Input: part model. Units: mm. Frame: model coordinates. A direction names the side the tool comes from. Round coordinates to 2 decimals unless told otherwise and drop trailing zeros. Loops run counter-clockwise (first coordinate to the right, second up) from the corner with the lowest first, then second, coordinate; pieces in that order, holes last. Notation, with made-up numbers: M -14.75,16 L 43.25,16 A16 ccw 43.25,20 Z; hole C 53.5,-21 d11. An arc over 180 degrees is marked long. Put each result on its own line as item: value. Start each with the question number.
1) Draft query along X for faces 6 (the face through (-1.5, -3, 0)), 7 (the face through (13, 4, -3)), 8 (the face through (21.4, -0.2, -0.5)). Return one class per face: +X half, -X half, draft (parallel to the pull), parting line (faces both ways), or undercut.
2) Line query: probe 1 along X at (y, z) = (-4.75, 3); probe 2 along X at (y, z) = (-1, -3); probe 3 along X at (y, z) = (8.75, -2.25). Output: solid intervals per line, ascending.
3) Section A-A on y = -1.3. State how many separate pieces and enclosed holes the cut face has, plus the area to 3 significant figures.
4) Section D-D on z = 4.75. Output: boundary loops of the cut face in (x, y).
5) Section C-C on z = 0.5. Output: boundary loops of the cut face in (x, y), plus the area to 3 significant figures.
6) Section B-B on x = 18.5. Output: boundary loops of the cut face in (y, z).
7) Reachability of faces 1 (the face through (0, -6, 4)), 2 (the face through (-6.2, -3, 0)), 3 (the face through (0, 10, -4)), 4 (the face through (19, 3.4, 3)), 5 (the face through (-9, 0, 0)) from +Z, -Z, +X, -X, +Y, -Y: full face, straight path, thin tool, end or side. Return the list, or none.
8) Pin query (flat end, axial travel): pin 1 (3.5 mm diameter, centred on y = 1.5, z = -2.5, fed in from +X); pin 2 (6.5 mm diameter, centred on y = -4, z = -1.5, fed in from +X); pin 3 (2.5 mm diameter, centred on x = 2.5, z = -1, fed in from +Y); pin 4 (2.5 mm diameter, centred on x = 20, y = -3, fed in from -Z). Return the tip coordinate at first contact, or that it passes through.
from build123d import *

# Parameters (mm, degrees)
SKETCH2_W           = 26
SKETCH2_H           = 11
SKETCH2_W_2         = 20.4
SKETCH2_H_2         = 6.5
BOSS_EXTRUDE1_DEPTH = 10
SKETCH3_W           = 26
SKETCH3_H           = 11
SKETCH3_W_2         = 2.5
SKETCH3_H_2         = 6.5
BOSS_EXTRUDE2_DEPTH = 6
SKETCH4_W           = 11
SKETCH4_H           = 9.4
SKETCH4_R           = 2.85
BOSS_EXTRUDE3_DEPTH = 6
FILLET1_R           = 2


with BuildPart() as part:
    # Sketch2 → Boss-Extrude1 (new body)
    with BuildSketch(Plane(origin=(0, 0, 0), x_dir=(1, 0, 0), z_dir=(0, 1, 0))):
        Rectangle(SKETCH2_W, SKETCH2_H)
        Rectangle(SKETCH2_W_2, SKETCH2_H_2, mode=Mode.SUBTRACT)
    extrude(amount=BOSS_EXTRUDE1_DEPTH)

    # Sketch3 → Boss-Extrude2 (add)
    with BuildSketch(Plane.XZ):
        Rectangle(SKETCH3_W, SKETCH3_H)
        with Locations((-7.45, 0)):
            Rectangle(SKETCH3_W_2, SKETCH3_H_2, mode=Mode.SUBTRACT)
        with Locations((-0.25, 0)):
            Rectangle(SKETCH3_W_2, SKETCH3_H_2, mode=Mode.SUBTRACT)
        with Locations((7.45, 0)):
            Rectangle(SKETCH3_W_2, SKETCH3_H_2, mode=Mode.SUBTRACT)
    extrude(amount=BOSS_EXTRUDE2_DEPTH)

    # Sketch4 → Boss-Extrude3 (add)
    # profile 1 of 2: a face of its own
    with BuildSketch(Plane.XY.offset(5.5)):
        with Locations((18.5, -1.3)):
            Rectangle(SKETCH4_W, SKETCH4_H)
        with Locations((18.5, -1.3)):
            Circle(SKETCH4_R, mode=Mode.SUBTRACT)
    # profile 2 of 2: a face of its own
    with BuildSketch(Plane.XY.offset(5.5)):
        with Locations((-18.5, -1.3)):
            Rectangle(SKETCH4_W, SKETCH4_H)
        with Locations(Location((-18.5, -1.3, 0), (0, 0, 180))):
            Circle(SKETCH4_R, mode=Mode.SUBTRACT)
    extrude(amount=-BOSS_EXTRUDE3_DEPTH)

    # Fillet1
    fillet1_edges = [part.edges().sort_by_distance(p)[0] for p in [
        (13, -1.3, -0.5),
        (13, 3.4, 2.5),
        (-13, -1.3, -0.5),
        (-13, 3.4, 2.5),
    ]]
    fillet(fillet1_edges, radius=FILLET1_R)


solid = part.part
Geometry results:
1. face 6: undercut
1. face 7: +X half
1. face 8: draft
2. probe 1: x = -24 to -8.7, -6.2 to -1.5, 1 to 6.2, 8.7 to 24
2. probe 2: x = -13 to -8.7, -6.2 to -1.5, 1 to 6.2, 8.7 to 13
2. probe 3: x = -13 to -10.2, 10.2 to 13
3. separate pieces: 3
3. enclosed holes: 3
3. area: 303 mm²
4. outline: M -24,-6 L 24,-6 L 24,3.4 L 15,3.4 A2 cw 13,5.4 L 13,10 L -13,10 L -13,5.4 A2 cw -15,3.4 L -24,3.4 Z; hole C -18.5,-1.3 d5.7; hole C 18.5,-1.3 d5.7
5. outline: M -24,-6 L -8.7,-6 L -8.7,0 L -10.2,0 L -10.2,10 L -13,10 L -13,5.4 A2 cw -15,3.4 L -24,3.4 Z; M -6.2,-6 L -1.5,-6 L -1.5,0 L -6.2,0 Z; M 1,-6 L 6.2,-6 L 6.2,0 L 1,0 Z; M 8.7,-6 L 24,-6 L 24,3.4 L 15,3.4 A2 cw 13,5.4 L 13,10 L 10.2,10 L 10.2,0 L 8.7,0 Z; hole C -18.5,-1.3 d5.7; hole C 18.5,-1.3 d5.7
5. area: 324 mm²
6. outline: M -6,-0.5 L -4.15,-0.5 L -4.15,5.5 L -6,5.5 Z; M 1.55,-0.5 L 3.4,-0.5 L 3.4,5.5 L 1.55,5.5 Z
7. face 1: +Z, -Z, +X, -X, -Y
7. face 2: +Y, -Y
7. face 3: +Z, -Z, +X, -X, +Y
7. face 4: +Z, -Z, +X, +Y
7. face 5: +Y
8. pin 1: stops at x = 14.03
8. pin 2: stops at x = 24
8. pin 3: stops at y = 0
8. pin 4: stops at z = -0.5
